```python
from build123d import *

# Parameters (mm, degrees)
SKETCH1_R           = 2
SKETCH1_R_2         = 10
BOSS_EXTRUDE1_DEPTH = 6
SKETCH2_W           = 50
SKETCH2_H           = 5.1
CUT_EXTRUDE1_DEPTH  = 299.24484337


with BuildPart() as part:
    # Sketch1 → Boss-Extrude1 (new body)
    with BuildSketch(Plane(origin=(0, 0, 0), x_dir=(1, 0, 0), z_dir=(0, 1, 0))):
        with BuildLine():
            Line((42.467703605, -75), (-167.432296395, -75))
            Line((-167.432296395, -75), (-167.432296395, -69.9))
            Line((-167.432296395, -69.9), (-172.532296395, -69.9))
            Line((-172.532296395, -69.9), (-172.532296395, -75))
            Line((-172.532296395, -75), (-192.532296395, -75))
            Line((-192.532296395, -75), (-192.532296395, -69.9))
            Line((-192.532296395, -69.9), (-197.632296395, -69.9))
            Line((-197.632296395, -69.9), (-197.632296395, -75))
            Line((-197.632296395, -75), (-257.532296395, -75))
            ThreePointArc((-257.532296395, -75), (-272.321614297, -56.461299938), (-282.622205976, -35.1))
            Line((-282.622205976, -35.1), (-272.622205976, -35.1))
            Line((-272.622205976, -35.1), (-272.622205976, -30))
            Line((-272.622205976, -30), (-284.267246142, -30))
            ThreePointArc((-284.267246142, -30), (-288.598313573, 0), (-284.267246142, 30))
            Line((-284.267246142, 30), (-272.622205976, 30))
            Line((-272.622205976, 30), (-272.622205976, 35.1))
            Line((-272.622205976, 35.1), (-282.622205976, 35.1))
            ThreePointArc((-282.622205976, 35.1), (-272.321614297, 56.461299938), (-257.532296395, 75))
            Line((-257.532296395, 75), (-197.632296395, 75))
            Line((-197.632296395, 75), (-197.632296395, 69.9))
            Line((-197.632296395, 69.9), (-192.532296395, 69.9))
            Line((-192.532296395, 69.9), (-192.532296395, 75))
            Line((-192.532296395, 75), (-172.532296395, 75))
            Line((-172.532296395, 75), (-172.532296395, 69.9))
            Line((-172.532296395, 69.9), (-167.432296395, 69.9))
            Line((-167.432296395, 69.9), (-167.432296395, 75))
            Line((-167.432296395, 75), (42.467703605, 75))
            Line((42.467703605, 75), (42.467703605, -75))
        make_face()
        with Locations(Location((-52.532296395, 67, 0), (0, 0, 270))):
            Circle(SKETCH1_R, mode=Mode.SUBTRACT)
        with Locations(Location((-22.532296395, 67, 0), (0, 0, 270))):
            Circle(SKETCH1_R, mode=Mode.SUBTRACT)
        with Locations(Location((-22.532296395, 43, 0), (0, 0, 270))):
            Circle(SKETCH1_R, mode=Mode.SUBTRACT)
        with Locations(Location((-52.532296395, 43, 0), (0, 0, 270))):
            Circle(SKETCH1_R, mode=Mode.SUBTRACT)
        with Locations(Location((-22.532296395, -67, 0), (0, 0, 90))):
            Circle(SKETCH1_R, mode=Mode.SUBTRACT)
        with Locations(Location((-22.532296395, -43, 0), (0, 0, 90))):
            Circle(SKETCH1_R, mode=Mode.SUBTRACT)
        with Locations(Location((-52.532296395, -43, 0), (0, 0, 90))):
            Circle(SKETCH1_R, mode=Mode.SUBTRACT)
        with Locations(Location((-52.532296395, -67, 0), (0, 0, 90))):
            Circle(SKETCH1_R, mode=Mode.SUBTRACT)
        with Locations(Location((-86.761151279, 0, 0), (0, 0, 270))):
            Circle(SKETCH1_R_2, mode=Mode.SUBTRACT)
        with Locations(Location((-235.692156702, 0, 0), (0, 0, 270))):
            Circle(SKETCH1_R_2, mode=Mode.SUBTRACT)
    extrude(amount=BOSS_EXTRUDE1_DEPTH)

    # Sketch2 → Cut-Extrude1 (cut, through all)
    with BuildSketch(Plane(origin=(0, 6, 0), x_dir=(1, 0, 0), z_dir=(0, 1, 0))):
        with Locations((-32.532296395, 22.55)):
            Rectangle(SKETCH2_W, SKETCH2_H)
        with Locations((-32.532296395, -22.55)):
            Rectangle(SKETCH2_W, SKETCH2_H)
    extrude(amount=-CUT_EXTRUDE1_DEPTH, mode=Mode.SUBTRACT)


solid = part.part
```
Can you work these out from the model? Positions are in its coordinate system, mm. A direction names the side the tool comes from. Round coordinates to 2 decimals unless told otherwise and drop trailing zeros. Loops run counter-clockwise (first coordinate to the right, second up) from the corner with the lowest first, then second, coordinate; pieces in that order, holes last. Notation, with made-up numbers: M -3.5,-15 L 41.5,-15 A31 ccw 41.5,11 Z; hole C 43,27.25 d3. An arc over 180 degrees is marked long. Answer in a Markdown table with one row per item.
1. On a 3-axis mill with a long thin cutter (end or side, diameter ignored), from which of +Z, -Z, +X, -X, +Y, -Y can I reach the whole of each face in a straight line? I mean faces 1 (the face through (-33, 3, 25.1)), 2 (the face through (-278, 3, 35.1)), 3 (the face through (-272.144, 2.958, 56.743)). Say none if no direction works.
Established:
| item | result |
|---|---|
| face 1 | +Y, -Y |
| face 2 | -X, +Y, -Y |
| face 3 | +Z, -X, +Y, -Y |
2. If we section it at D-D, the plane z = 62: Please give me the cut outline in (x, y), plus the area to 3 significant figures.
Established:
| item | result |
|---|---|
| outline | M -268.59,0 L 42.47,0 L 42.47,6 L -268.59,6 Z |
| area | 1,870 mm² |
3. If we section it at C-C, the plane z = -53: Please give me the cut outline in (x, y).
Established:
| item | result |
|---|---|
| outline | M -274.41,0 L 42.47,0 L 42.47,6 L -274.41,6 Z |
4. If we section it at A-A, the plane z = 0: Please give me the cut outline in (x, y).
Established:
| item | result |
|---|---|
| outline | M -288.6,0 L -245.69,0 L -245.69,6 L -288.6,6 Z; M -225.69,0 L -96.76,0 L -96.76,6 L -225.69,6 Z; M -76.76,0 L 42.47,0 L 42.47,6 L -76.76,6 Z |
5. If we section it at B-B, the plane y = 1: Give the number of separate pieces and of enclosed holes in the cut face, plus the area to 3 significant figures.
Established:
| item | result |
|---|---|
| separate pieces | 1 |
| enclosed holes | 12 |
| area | 46,800 mm² |
6. I'm going to push flat-ended pins straight in: pin 1 Ø3 at (x, y) = (-278.5, 4) entering from -Z; pin 2 Ø1.5 at (y, z) = (4, -32) entering from -X; pin 3 Ø2.5 at (y, z) = (2.5, -73.5) entering from -X. Where does each tip first touch, or does it pass through?
Established:
| item | result |
|---|---|
| pin 1 | z = -48.23 |
| pin 2 | x = -272.62 |
| pin 3 | x = -260.18 |
7. Please list where these lines run through material, in increasing order: line 1 (Z direction, x = -26, y = 3.45); line 2 (Z direction, x = -87, y = 5.4); line 3 (X direction, y = 3.4, z = 67). Write a range as from..to.
Established:
| item | result |
|---|---|
| line 1 | -75..-25.1, -20..20, 25.1..75 |
| line 2 | -75..-10, 10..75 |
| line 3 | -264.76..-54.53, -50.53..-24.53, -20.53..42.47 |
